Geometry: final body of the model. Coordinates: model frame, mm. A direction names the side the tool comes from. Give positions to 0.01 mm unless a question says otherwise; leave off trailing zeros. Write each loop counter-clockwise with the first axis right and the second up, starting at its lowest first coordinate (ties: lowest second). Pieces come first, ordered by that corner, then holes. Notation, with made-up numbers: M 62.25,63.25 L 95.25,63.25 A7 ccw 95.25,75.25 Z; hole C -19,89.5 d5. An arc over 180 degrees is marked long. Answer as a JSON object with one key per item and string values.
Autodesk Inventor part; units mm, degrees
ref_plane "YZ Plane" through (0, 0, 0) normal (1, 0, 0) x (0, 1, 0)
ref_plane "XZ Plane" through (0, 0, 0) normal (0, 1, 0) x (-1, 0, 0)
ref_plane "XY Plane" through (0, 0, 0) normal (0, 0, 1) x (1, 0, 0)
sketch "Sketch1" plane through (0, 0, 0) normal (0, 1, 0) x (-1, 0, 0)
  line L0 (6, 8) -> (-6, 8)
  line L1 (-8, 6) -> (-8, -6)
  line L2 (-6, -8) -> (6, -8)
  line L3 (8, -6) -> (8, 6)
  arc A0 (8, 6) -> (6, 8) centre (6, 6) ccw
  arc A1 (-6, 8) -> (-8, 6) centre (-6, 6) ccw
  arc A2 (-8, -6) -> (-6, -8) centre (-6, -6) ccw
  arc A3 (6, -8) -> (8, -6) centre (6, -6) ccw
  point P0 (0, 0)
  point P1 (8, 8)
  point P2 (-8, 8)
  point P3 (8, -8)
  dimension "d0" = 16
  dimension "d1" = 16
  dimension "d2" = 8
  dimension "d3" = 8
  dimension "d4" = 2
extrude "Extrusion1" add sketch "Sketch1" along normal blind 43
sketch "Sketch2" plane through (0, 0, 0) normal (0, -1, 0) x (1, 0, 0)
  line L0 (-6, 5.875) -> (-6, 3.125) construction
  line L1 (-7.375, 5.875) -> (-7.375, 3.125)
  line L2 (-4.625, 3.125) -> (-4.625, 5.875)
  arc A0 (-4.625, 5.875) -> (-7.375, 5.875) centre (-6, 5.875) ccw
  arc A1 (-7.375, 3.125) -> (-4.625, 3.125) centre (-6, 3.125) ccw
  line L3 (6, -3.125) -> (6, -5.875) construction
  line L4 (4.625, -3.125) -> (4.625, -5.875)
  line L5 (7.375, -5.875) -> (7.375, -3.125)
  arc A2 (7.375, -3.125) -> (4.625, -3.125) centre (6, -3.125) ccw
  arc A3 (4.625, -5.875) -> (7.375, -5.875) centre (6, -5.875) ccw
  point P0 (0, 0)
  point P1 (0, 0)
  point P2 (-6, 4.5)
  point P3 (6, -4.5)
  dimension "d7" = 2.75
  dimension "d8" = 12
  dimension "d9" = 6
  dimension "d10" = 9
  dimension "d11" = 4.5
  dimension "d12" = 2.75
  dimension "d13" = 2.75
  dimension "d14" = 2.75
extrude "Extrusion2" cut sketch "Sketch2" against normal blind 2.5
hole "Hole1" at (0, 0, 0) direction (0, 1, 0) diameter 6.756 end through all
sketch "Sketch3" plane through (0, 43, 0) normal (0, 1, 0) x (1, 0, 0)
  line L0 (-6, 1.5) -> (-6, -1.5) construction
  line L1 (-6.65, 1.5) -> (-6.65, -1.5)
  line L2 (-5.35, -1.5) -> (-5.35, 1.5)
  arc A0 (-5.35, 1.5) -> (-6.65, 1.5) centre (-6, 1.5) ccw
  arc A1 (-6.65, -1.5) -> (-5.35, -1.5) centre (-6, -1.5) ccw
  line L3 (6, 1.5) -> (6, -1.5) construction
  line L4 (5.35, 1.5) -> (5.35, -1.5)
  line L5 (6.65, -1.5) -> (6.65, 1.5)
  arc A2 (6.65, 1.5) -> (5.35, 1.5) centre (6, 1.5) ccw
  arc A3 (5.35, -1.5) -> (6.65, -1.5) centre (6, -1.5) ccw
  line L6 (-6, 0) -> (6, 0) construction
  line L7 (6, 8) -> (-6, 8)
  point P0 (0, 0)
  dimension "d25" = 0.65
  dimension "d26" = 0.65
  dimension "d27" = 3
  dimension "d29" = 0
  dimension "d30" = 12
  dimension "d31" = 6
  dimension "d32" = 3
extrude "Extrusion3" add sketch "Sketch3" along normal blind 1.5
equation "\"d12\" = d7"
equation "\"d13\" = d7"
equation "\"d14\" = d7"
equation "\"d26\" = d25"
equation "\"d27\" = d32"
properties part number "Camera Mount 30mm"
1) Contact query for flat-ended pins moving along their axis: P1, Ø2, axis at x = -0.5, z = 2.5, coming from the +Y side; P2, Ø1.6, axis at y = 43.5, z = -0.5, coming from the +X side; P3, Ø1.2, axis at y = 44, z = -0.5, coming from the -X side; P4, Ø4, axis at x = 0, z = 0, coming from the +Y side. Output: stop coordinate, or through.
Geometry check:
{"P1": "stops at y = 43", "P2": "stops at x = 8", "P3": "stops at x = -6.65", "P4": "passes through"}
2) Cut plane C-C on x = -0.5. Return loops of the section in (y, z), and give its area (3 significant figures).
Geometry check:
{"outline": "M 0,-8 L 43,-8 L 43,-3.34 L 0,-3.34 Z; M 0,3.34 L 43,3.34 L 43,8 L 0,8 Z", "area": "401 mm2"}
3) Pull-direction query (Z, two-part tool) for faces 1 (the flat face through (0, 0, 4)), 2 (the flat face through (6, 2.5, -4)), 3 (the cylindrical face through (-6.01, 43.74, -2.15)), 4 (the cylindrical face through (7.43, 21.2, 7.4)); classes: pulls with the +Z half, pulls with the -Z half, needs draft (parallel to the pull), parting line crosses it, or undercut.
Geometry check:
{"face 1": "needs draft", "face 2": "undercut", "face 3": "pulls with the -Z half", "face 4": "pulls with the +Z half"}
4) Cut plane D-D on z = 4. Return loops of the section in (x, y) (3 decimals).
Geometry check:
{"outline": "M -8,0 L -7.375,0 L -7.375,2.5 L -4.625,2.5 L -4.625,0 L 8,0 L 8,43 L -8,43 Z"}
5) Set-up query: faces 5 (the cylindrical face through (-5.99, 43.74, 2.15)), 6 (the flat face through (8, 21, 0)), 7 (the flat face through (0, 21, 8)), 8 (the flat face through (-6, 2.5, 5)), 9 (the flat face through (5.35, 44, 0)). Return all of +Z, -Z, +X, -X, +Y, -Y with unobstructed straight access to the full face (end or side cutting, diameter ignored); none if empty.
Geometry check:
{"face 5": "+Z, +Y", "face 6": "+Z, -Z, +X, +Y, -Y", "face 7": "+Z, +X, -X, +Y, -Y", "face 8": "-Y", "face 9": "+Z, -Z, +Y"}
6) Cut plane A-A on z = 0. Return loops of the section in (x, y).
Geometry check:
{"outline": "M -8,0 L -3.38,0 L -3.38,43 L -5.35,43 L -5.35,44.5 L -6.65,44.5 L -6.65,43 L -8,43 Z; M 3.38,0 L 8,0 L 8,43 L 6.65,43 L 6.65,44.5 L 5.35,44.5 L 5.35,43 L 3.38,43 Z"}
7) Line query: line 1 (X direction, y = 18.5, z = 0); line 2 (Y direction, x = 0.25, z = -4.25). Output: solid intervals per line, ascending. Write a range as from..to.
Geometry check:
{"line 1": "x = -8..-3.38, 3.38..8", "line 2": "y = 0..43"}
8) Cut plane B-B on y = 10.5. Return loops of the section in (x, z).
Geometry check:
{"outline": "M -8,-6 A2 ccw -6,-8 L 6,-8 A2 ccw 8,-6 L 8,6 A2 ccw 6,8 L -6,8 A2 ccw -8,6 Z; hole C 0,0 d6.76"}
